```python
from build123d import *

# Parameters (mm, degrees)
F0_W     = 20
F0_H     = 20
F1_DEPTH = 20
F3_DEPTH = 1


with BuildPart() as f1:
    # F0 (on Front) → F1 (new body)
    with BuildSketch(Plane.XZ):
        with Locations((-10, -10)):
            Rectangle(F0_W, F0_H)
    extrude(amount=F1_DEPTH)

    # F2 (on face) → F3 (cut)
    with BuildSketch(Plane(origin=(0, 0, -20), x_dir=(1, 0, 0), z_dir=(0, 0, -1))):
        with BuildLine():
            ThreePointArc((-13.0285681023, 6.9714318977), (-16.2748573364, 6.9714318977), (-16.2748573364, 3.7251426636))
            Line((-16.2748573364, 3.7251426636), (-13.0285681023, 6.9714318977))
        make_face()
        with BuildLine():
            ThreePointArc((-16.9547054218, 16.9547054218), (-16.9547054218, 13.2777501596), (-13.2777501596, 13.2777501596))
            Line((-13.2777501596, 13.2777501596), (-16.9547054218, 16.9547054218))
        make_face()
        with BuildLine():
            Line((-16.9547054218, 16.9547054218), (-13.2777501596, 13.2777501596))
            ThreePointArc((-13.2777501596, 13.2777501596), (-12.7141410062, 14.1212508666), (-12.5162277907, 15.1162277907))
            ThreePointArc((-12.5162277907, 15.1162277907), (-14.1212508666, 17.5183145752), (-16.9547054218, 16.9547054218))
        make_face()
        with BuildLine():
            ThreePointArc((-11.8384776311, 11.8384776311), (-12.6, 10), (-11.8384776311, 8.1615223689))
            Line((-11.8384776311, 8.1615223689), (-10, 10))
            Line((-10, 10), (-11.8384776311, 11.8384776311))
        make_face()
        with BuildLine():
            Line((-10, 10), (-11.8384776311, 8.1615223689))
            ThreePointArc((-11.8384776311, 8.1615223689), (-10, 7.4), (-8.1615223689, 8.1615223689))
            Line((-8.1615223689, 8.1615223689), (-10, 10))
        make_face()
        with BuildLine():
            Line((-13.0285681023, 6.9714318977), (-16.2748573364, 3.7251426636))
            ThreePointArc((-16.2748573364, 3.7251426636), (-13.7732731826, 3.2275466374), (-12.3562395882, 5.3482872806))
            ThreePointArc((-12.3562395882, 5.3482872806), (-12.5309720761, 6.2267268174), (-13.0285681023, 6.9714318977))
        make_face()
        with BuildLine():
            Line((-11.8384776311, 11.8384776311), (-10, 10))
            Line((-10, 10), (-8.1615223689, 11.8384776311))
            ThreePointArc((-8.1615223689, 11.8384776311), (-10, 12.6), (-11.8384776311, 11.8384776311))
        make_face()
        with BuildLine():
            Line((-8.1615223689, 11.8384776311), (-10, 10))
            Line((-10, 10), (-8.1615223689, 8.1615223689))
            ThreePointArc((-8.1615223689, 8.1615223689), (-7.5979132155, 9.0050230759), (-7.4, 10))
            ThreePointArc((-7.4, 10), (-7.5979132155, 10.9949769241), (-8.1615223689, 11.8384776311))
        make_face()
        with BuildLine():
            ThreePointArc((-7.4, 10), (-7.5979132155, 9.0050230759), (-8.1615223689, 8.1615223689))
            Line((-8.1615223689, 8.1615223689), (-6.7114877282, 6.7114877282))
            ThreePointArc((-6.7114877282, 6.7114877282), (-3.8780331729, 7.2750968816), (-2.2730100971, 4.8730100971))
            ThreePointArc((-2.2730100971, 4.8730100971), (-2.4709233125, 3.8780331729), (-3.034532466, 3.034532466))
            Line((-3.034532466, 3.034532466), (0, 0))
            Line((0, 0), (0, 20))
            Line((0, 20), (-3.3504526736, 16.6495473264))
            ThreePointArc((-3.3504526736, 16.6495473264), (-2.7868435202, 15.8060466194), (-2.5889303047, 14.8110696953))
            ThreePointArc((-2.5889303047, 14.8110696953), (-4.1939533806, 12.4089829107), (-7.0274079358, 12.9725920642))
            Line((-7.0274079358, 12.9725920642), (-8.1615223689, 11.8384776311))
            ThreePointArc((-8.1615223689, 11.8384776311), (-7.5979132155, 10.9949769241), (-7.4, 10))
        make_face()
        with BuildLine():
            ThreePointArc((-2.2730100971, 4.8730100971), (-3.8780331729, 7.2750968816), (-6.7114877282, 6.7114877282))
            Line((-6.7114877282, 6.7114877282), (-3.034532466, 3.034532466))
            ThreePointArc((-3.034532466, 3.034532466), (-2.4709233125, 3.8780331729), (-2.2730100971, 4.8730100971))
        make_face()
        with BuildLine():
            Line((-3.034532466, 3.034532466), (-6.7114877282, 6.7114877282))
            ThreePointArc((-6.7114877282, 6.7114877282), (-6.7114877282, 3.034532466), (-3.034532466, 3.034532466))
        make_face()
        with BuildLine():
            ThreePointArc((-3.3504526736, 16.6495473264), (-7.0274079358, 16.6495473264), (-7.0274079358, 12.9725920642))
            Line((-7.0274079358, 12.9725920642), (-3.3504526736, 16.6495473264))
        make_face()
        with BuildLine():
            Line((-3.3504526736, 16.6495473264), (-7.0274079358, 12.9725920642))
            ThreePointArc((-7.0274079358, 12.9725920642), (-4.1939533806, 12.4089829107), (-2.5889303047, 14.8110696953))
            ThreePointArc((-2.5889303047, 14.8110696953), (-2.7868435202, 15.8060466194), (-3.3504526736, 16.6495473264))
        make_face()
    extrude(amount=-F3_DEPTH, mode=Mode.SUBTRACT)


solid = f1.part
```
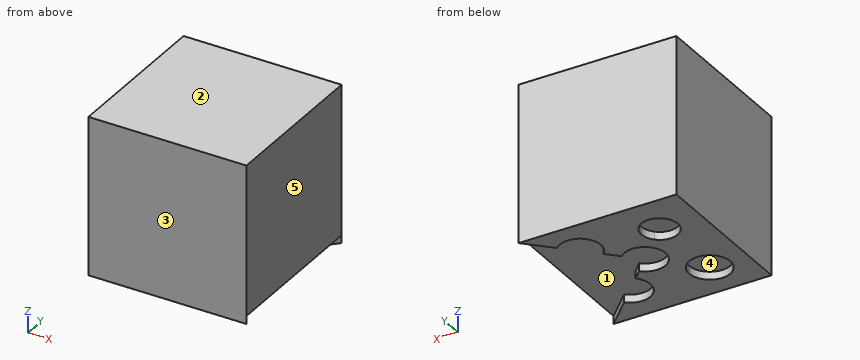
Geometry check sheet. Reference: the model listing, model coordinates, mm. Face numbers are marked on the shaded views. A direction names the side the tool comes from. Coordinates: 2 decimals unless noted, no trailing zeros. Order: outer loops, then holes, each group sorted by start corner. A loop starts at its lowest first (then second) coordinate and runs counter-clockwise, first axis right, second up. Notation, with made-up numbers: (73.5, -14) - (83.5, -14) arc R29 cw to (83.5, 14) - close; hole circle Ø7 at (88.5, -23). An arc over 180 degrees is marked (long way). Answer as a JSON object with one key per item and string values. Group by question number.
Item 1: Depth check by flat-ended pin: pin 1 Ø5 at (x, y) = (-5, -9) entering from -Z. Enter the tip coordinate at first touch or a pass-through.
Item 2: Scan line: probe 1 along Z at (x, y) = (-4.5, -8.25). Record every from-to range of solid material in increasing order.
Item 3: Sectioned sample at B-B, the plane y = -11. Record the cut outline in (x, z).
Item 4: Draft check along Y on the marked faces 1, 2 and 3. Enter one of: +Y half, -Y half, draft (parallel to the pull), parting line (faces both ways), or undercut.
Item 5: Sectioned sample at D-D, the plane y = -16.25. Record the cut outline in (x, z).
Item 6: Sectioned sample at A-A, the plane x = -2. Record the cut outline in (y, z), and give its area (3 significant figures).
Item 7: Tool access check on the marked faces 4 and 5. Record the directions out of +Z, -Z, +X, -X, +Y, -Y that give a thin tool (end or side, any length) a straight path to the whole face; none if there is none.
Item 8: Sectioned sample at C-C, the plane x = -5. Record the cut outline in (y, z), and give its area (3 significant figures).
Resolved:
{
 "1": {"pin 1": "z = -19"},
 "2": {"probe 1": "-19 to 0"},
 "3": {"outline": "(-20, -20) - (-12.4, -20) - (-12.4, -19) - (0, -19) - (0, 0) - (-20, 0) - close"},
 "4": {"face 1": "undercut", "face 2": "draft", "face 3": "-Y half"},
 "5": {"outline": "(-20, -20) - (-17.46, -20) - (-17.46, -19) - (-12.78, -19) - (-12.78, -20) - (-7.35, -20) - (-7.35, -19) - (0, -19) - (0, 0) - (-20, 0) - close"},
 "6": {"outline": "(-20, -20) - (-18, -20) - (-18, -19) - (-2, -19) - (-2, -20) - (0, -20) - (0, 0) - (-20, 0) - close", "area": "384 mm^2"},
 "7": {"face 4": "-Z", "face 5": "+Z, -Z, +X, +Y, -Y"},
 "8": {"outline": "(-20, -20) - (-17.4, -20) - (-17.4, -19) - (-2.28, -19) - (-2.28, -20) - (0, -20) - (0, 0) - (-20, 0) - close", "area": "385 mm^2"}
}
